Autodesk Inventor part; units mm, degrees
ref_plane "IP_1_XY" through (4, 0, 0) normal (1, 0, 0) x (0, 0, -1)
ref_plane "IP_1_YZ" through (4, 0, 0) normal (0, 0, -1) x (0, 1, 0)
ref_plane "IP_1_ZX" through (4, 0, 0) normal (0, 1, 0) x (1, 0, 0)
sketch "Sketch_1" plane through (0, 0, 0) normal (0, 0, 1) x (1, 0, 0)
  line L0 (7.3, 0) -> (0.7, 0)
  line L1 (0.7, 2.375) -> (7.3, 2.375)
  line L2 (7.3, 2.375) -> (7.3, 3.125)
  line L3 (7.3, 3.125) -> (0.7, 3.125)
  line L4 (0.7, 3.125) -> (0.7, 2.375)
revolve "Revolution1" add sketch "Sketch_1" angle 360 about axis through (7.3, 0, 0) along (1, 0, 0)
sketch "Sketch_2" plane through (0, 0, 0) normal (0, 0, 1) x (1, 0, 0)
  line L0 (6, 2.75) -> (2, 2.75)
  line L1 (2, 2.75) -> (2, 3.5)
  line L2 (2, 3.5) -> (6, 3.5)
  line L3 (6, 3.5) -> (6, 2.75)
  line L4 (6, 2.75) -> (2, 2.75)
revolve "Revolution2" cut sketch "Sketch_2" angle 360 about axis through (6, 2.75, 0) along (1, 0, 0)
pattern_linear "Rectangular Pattern1" count 3 spacing 2.75 along (0, -0.5, 0.866) count 3 spacing 2.75 along (0, -0.5, -0.866) of "Revolution2"
ref_plane "IP_1_XY" through (4, 0, 0) normal (1, 0, 0) x (0, 0, -1)
ref_plane "IP_1_YZ" through (4, 0, 0) normal (0, 0, -1) x (0, 1, 0)
ref_plane "IP_1_ZX" through (4, 0, 0) normal (0, 1, 0) x (1, 0, 0)
ref_plane "IP_3_1_XY" through (4, 2.75, 0) normal (1, 0, 0) x (0, 0, -1)
ref_plane "IP_3_1_YZ" through (4, 2.75, 0) normal (0, 0, -1) x (0, 1, 0)
ref_plane "IP_3_1_ZX" through (4, 2.75, 0) normal (0, 1, 0) x (1, 0, 0)
ref_plane "IP_3_2_XY" through (4, 1.375, 2.3816) normal (1, 0, 0) x (0, 0, -1)
ref_plane "IP_3_2_YZ" through (4, 1.375, 2.3816) normal (0, 0, -1) x (0, 1, 0)
ref_plane "IP_3_2_ZX" through (4, 1.375, 2.3816) normal (0, 1, 0) x (1, 0, 0)
ref_plane "IP_3_3_XY" through (4, -1.375, 2.3816) normal (1, 0, 0) x (0, 0, -1)
ref_plane "IP_3_3_YZ" through (4, -1.375, 2.3816) normal (0, 0, -1) x (0, 1, 0)
ref_plane "IP_3_3_ZX" through (4, -1.375, 2.3816) normal (0, 1, 0) x (1, 0, 0)
ref_plane "IP_3_4_XY" through (4, -2.75, 0) normal (1, 0, 0) x (0, 0, -1)
ref_plane "IP_3_4_YZ" through (4, -2.75, 0) normal (0, 0, -1) x (0, 1, 0)
ref_plane "IP_3_4_ZX" through (4, -2.75, 0) normal (0, 1, 0) x (1, 0, 0)
ref_plane "IP_3_5_XY" through (4, -1.375, -2.3816) normal (1, 0, 0) x (0, 0, -1)
ref_plane "IP_3_5_YZ" through (4, -1.375, -2.3816) normal (0, 0, -1) x (0, 1, 0)
ref_plane "IP_3_5_ZX" through (4, -1.375, -2.3816) normal (0, 1, 0) x (1, 0, 0)
ref_plane "IP_3_6_XY" through (4, 1.375, -2.3816) normal (1, 0, 0) x (0, 0, -1)
ref_plane "IP_3_6_YZ" through (4, 1.375, -2.3816) normal (0, 0, -1) x (0, 1, 0)
ref_plane "IP_3_6_ZX" through (4, 1.375, -2.3816) normal (0, 1, 0) x (1, 0, 0)
properties part number "HK0408FT2CA"
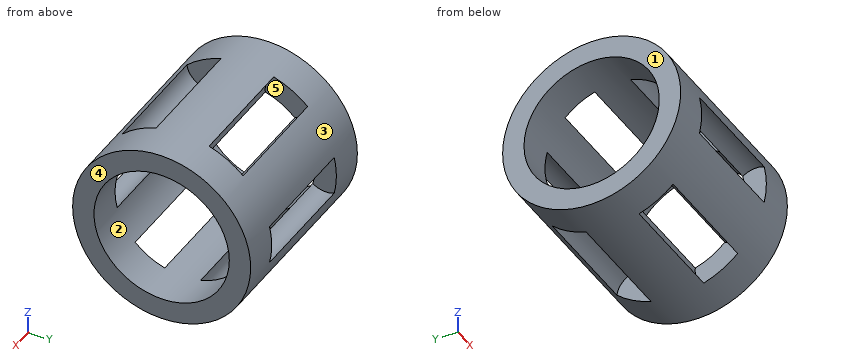
Here's how the part is built. I have some questions about the finished solid (model axes, mm). Face numbers are marked on the shaded views. A direction names the side the tool comes from. Coordinates: 2 decimals unless noted, no trailing zeros. Order: outer loops, then holes, each group sorted by start corner. A loop starts at its lowest first (then second) coordinate and runs counter-clockwise, first axis right, second up.
1) Which directions (+Z, -Z, +X, -X, +Y, -Y) give clear straight access to the entire face, cutting with the end or side of a thin tool? Please do the marked faces 4 and 5.
2) Imagine slicing it at D-D on z = -1.5. List the corners of the cut face in (x, y) for me.
3) Imagine slicing it at A-A on y = 0. List the corners of the cut face in (x, z) for me (3 decimals).
4) Imagine slicing it at C-C on x = 5.25. List the corners of the cut face in (y, z) for me (3 decimals), and give its area (3 significant figures).
5) I need wall thicknesses on line 1 (Z direction, x = 1.5, y = 0) (3 decimals); line 2 (X direction, y = 1, z = -2.5); line 3 (Y direction, x = 3, z = -2). Which ranges of each line are inside material? Lowest first, please.
6) We'd pull the mould along Y, two halves only. Please class the marked faces 1, 2 and 3: +Y half, -Y half, draft (parallel to the pull), parting line (faces both ways), or undercut.
7) Will these pins go through, and if not, where does the flat tip stop? pin 1 (2 mm diameter, centred on y = 2, z = 0.5, fed in from -X); pin 2 (2 mm diameter, centred on y = -0.5, z = -0.5, fed in from +X).
8) Imagine slicing it at B-B on z = 0. List the corners of the cut face in (x, y) for me (3 decimals), and give its area (3 significant figures).
Response values:
1. face 4: +Z, -Z, +X, +Y, -Y
1. face 5: none
2. outline: (0.7, -2.74) - (7.3, -2.74) - (7.3, -1.84) - (0.7, -1.84) - close; (0.7, 1.84) - (7.3, 1.84) - (7.3, 2.74) - (0.7, 2.74) - close
3. outline: (0.7, -3.125) - (7.3, -3.125) - (7.3, -2.375) - (0.7, -2.375) - close; (0.7, 2.375) - (7.3, 2.375) - (7.3, 3.125) - (0.7, 3.125) - close
4. outline: (-3.048, -0.688) arc R3.125 ccw to (-2.12, -2.296) arc R0.75 cw to (-1.668, -1.691) arc R2.375 cw to (-2.298, -0.599) arc R0.75 cw to start; (-3.048, 0.688) arc R0.75 cw to (-2.298, 0.599) arc R2.375 cw to (-1.668, 1.691) arc R0.75 cw to (-2.12, 2.296) arc R3.125 ccw to start; (-0.928, -2.984) arc R3.125 ccw to (0.928, -2.984) arc R0.75 cw to (0.631, -2.29) arc R2.375 cw to (-0.631, -2.29) arc R0.75 cw to start; (-0.928, 2.984) arc R0.75 cw to (-0.631, 2.29) arc R2.375 cw to (0.631, 2.29) arc R0.75 cw to (0.928, 2.984) arc R3.125 ccw to start; (1.668, -1.691) arc R0.75 cw to (2.12, -2.296) arc R3.125 ccw to (3.048, -0.688) arc R0.75 cw to (2.298, -0.599) arc R2.375 cw to start; (1.668, 1.691) arc R2.375 cw to (2.298, 0.599) arc R0.75 cw to (3.048, 0.688) arc R3.125 ccw to (2.12, 2.296) arc R0.75 cw to start
4. area: 6.49 mm2
5. line 1: z = -3.125 to -2.375, 2.375 to 3.125
5. line 2: x = 0.7 to 2, 6 to 7.3
5. line 3: y = -2.4 to -2.02, 2.02 to 2.4
6. face 1: draft
6. face 2: undercut
6. face 3: parting line
7. pin 1: stops at x = 0.7
7. pin 2: passes through
8. outline: (0.7, -3.125) - (2, -3.125) - (2, -2.375) - (0.7, -2.375) - close; (0.7, 2.375) - (2, 2.375) - (2, 3.125) - (0.7, 3.125) - close; (6, -3.125) - (7.3, -3.125) - (7.3, -2.375) - (6, -2.375) - close; (6, 2.375) - (7.3, 2.375) - (7.3, 3.125) - (6, 3.125) - close
8. area: 3.90 mm2
